Could you check a few things on this model? Use its own coordinates, in mm. A direction names the side the tool comes from. Coordinates: 2 decimals unless noted, no trailing zeros. Loops run counter-clockwise (first coordinate to the right, second up) from the corner with the lowest first, then second, coordinate; pieces in that order, holes last. Notation, with made-up numbers: (-33.75, 82.25) - (12.25, 82.25) arc R22 cw to (12.25, 121.25) - close; hole circle Ø9 at (28.5, 24). An arc over 180 degrees is marked (long way). Use CSV: the item, a comma, the result in double quotes.
from build123d import *

# Parameters (mm, degrees)
CYLINDER001_R           = 0.55
CYLINDER001_DEPTH       = 3.5
CYLINDER_R              = 1.1
CYLINDER_DEPTH          = 3.5
CUBE003_W               = 4
CUBE003_H               = 6
CUBE003_DEPTH           = 9
CUBE003_PLACEMENT_ANGLE = 15
CUBE002_W               = 4
CUBE002_H               = 6
CUBE002_DEPTH           = 8
CUBE002_PLACEMENT_ANGLE = 15
CUBE001_W               = 1.27
CUBE001_H               = 3
CUBE001_DEPTH           = 4
CUBE_W                  = 2.54
CUBE_H                  = 6.2
CUBE_DEPTH              = 8.2


with BuildPart() as cylinder001:
    # cylinder001 → cylinder001 (new body)
    with BuildSketch(Plane(origin=(1.27, 3.1, -3.5), x_dir=(1, 0, 0), z_dir=(0, 0, 1))):
        Circle(CYLINDER001_R)
    extrude(amount=CYLINDER001_DEPTH)


with BuildPart() as cylinder:
    # cylinder → cylinder (new body)
    with BuildSketch(Plane(origin=(1.27, 3.1, 5), x_dir=(1, 0, 0), z_dir=(0, 0, 1))):
        Circle(CYLINDER_R)
    extrude(amount=CYLINDER_DEPTH)


with BuildPart() as cube003:
    # cube003 → cube003 (new body)
    with BuildSketch(Plane.XY):
        with Locations((2, 3)):
            Rectangle(CUBE003_W, CUBE003_H)
    extrude(amount=CUBE003_DEPTH)


with BuildPart() as cube003_1:
    # cube003 placement: moved
    add(cube003.part.moved(Location((-1, -7.244444, 1.941143))).rotate(Axis((-1, -7.244444, 1.941143), (-1, 0, 0)), CUBE003_PLACEMENT_ANGLE))


with BuildPart() as cube002:
    # cube002 → cube002 (new body)
    with BuildSketch(Plane.XY):
        with Locations((2, 3)):
            Rectangle(CUBE002_W, CUBE002_H)
    extrude(amount=CUBE002_DEPTH)


with BuildPart() as cube002_1:
    # cube002 placement: moved
    add(cube002.part.moved(Location((-1, 6.761481, 1.811733))).rotate(Axis((-1, 6.761481, 1.811733), (1, 0, 0)), CUBE002_PLACEMENT_ANGLE))


with BuildPart() as cube001:
    # cube001 → cube001 (new body)
    with BuildSketch(Plane(origin=(0.635, -1, 1), x_dir=(1, 0, 0), z_dir=(0, 0, 1))):
        with Locations((0.635, 1.5)):
            Rectangle(CUBE001_W, CUBE001_H)
    extrude(amount=CUBE001_DEPTH)


with BuildPart() as group:
    # cube → cube (new body)
    with BuildSketch(Plane.XY):
        with Locations((1.27, 3.1)):
            Rectangle(CUBE_W, CUBE_H)
    extrude(amount=CUBE_DEPTH)

    # difference: cut cube001
    add(cube001.part, mode=Mode.SUBTRACT)

    # difference001: cut cube002
    add(cube002_1.part, mode=Mode.SUBTRACT)

    # difference002: cut cube003
    add(cube003_1.part, mode=Mode.SUBTRACT)

    # difference003: cut cylinder
    add(cylinder.part, mode=Mode.SUBTRACT)

    # Group: union cylinder001
    add(cylinder001.part)


solid = group.part
(1) Suppose I cut it at A-A (y = 1). Write out the boundary of the cut face in (x, z) (3 decimals), plus the area to 3 significant figures.
Computed:
outline,"(0, 0) - (2.54, 0) - (2.54, 8.2) - (0, 8.2) - close; hole (0.635, 1) - (1.905, 1) - (1.905, 5) - (0.635, 5) - close"
area,"15.7 mm²"
(2) Will these pins go through, and if not, where does the flat tip stop? pin 1 (1.5 mm diameter, centred on x = 0.5, y = 1, fed in from -Z); pin 2 (0.7 mm diameter, centred on x = 1, y = 3.5, fed in from +Z).
Computed:
pin 1,"stops at z = 0"
pin 2,"stops at z = 5"
(3) Thinking about a two-plate mould opening in X: for faces 1 (the face through (1.252, 5.633, 6.024)), 2 (the face through (0, 3, 4)), 3 (the face through (1, 1, 1)), which applies, +X half, -X half, draft (parallel to the pull), parting line (faces both ways), or undercut?
Computed:
face 1,"draft"
face 2,"-X half"
face 3,"undercut"
(4) Suppose I cut it at D-D (x = 1.1). Write out the boundary of the cut face in (y, z).
Computed:
outline,"(0, 0) - (2.58, 0) - (2.58, -3.5) - (3.62, -3.5) - (3.62, 0) - (6.2, 0) - (6.2, 3.91) - (5.05, 8.2) - (4.19, 8.2) - (4.19, 5) - (2.01, 5) - (2.01, 8.2) - (0.64, 8.2) - (0, 5.8) - (0, 5) - (2, 5) - (2, 1) - (0, 1) - close"
(5) Suppose I cut it at B-B (y = 3.1). Write out the boundary of the cut face in (x, z), plus the area to 3 significant figures.
Computed:
outline,"(0, 0) - (0.72, 0) - (0.72, -3.5) - (1.82, -3.5) - (1.82, 0) - (2.54, 0) - (2.54, 8.2) - (2.37, 8.2) - (2.37, 5) - (0.17, 5) - (0.17, 8.2) - (0, 8.2) - close"
area,"17.6 mm²"
(6) Which directions (+Z, -Z, +X, -X, +Y, -Y) give clear straight access to the entire face, cutting with the end or side of a thin tool? Please do faces 4 (the face through (1, 6.2, 2)), 5 (the face through (1.57, 3.56, -1.77)), 6 (the face through (1.032, 2.026, 6.578)), 7 (the face through (1, 1, 5)).
Computed:
face 4,"+Z, -Z, +X, -X, +Y"
face 5,"-Z"
face 6,"+Z"
face 7,"-Y"
(7) Suppose I cut it at C-C (z = 3). Write out the boundary of the cut face in (x, y) (3 decimals), plus the area to 3 significant figures.
Computed:
outline,"(0, 0) - (0.635, 0) - (0.635, 2) - (1.905, 2) - (1.905, 0) - (2.54, 0) - (2.54, 6.2) - (0, 6.2) - close"
area,"13.2 mm²"
(8) Please list where these lines run through material, in increasing order: line 1 (Z direction, x = 1.25, y = 1.5); line 2 (X direction, y = 3.1, z = 5.9); line 3 (X direction, y = 0.5, z = 4.5) (3 decimals).
Computed:
line 1,"z = 0 to 1, 5 to 8.2"
line 2,"x = 0 to 0.17, 2.37 to 2.54"
line 3,"x = 0 to 0.635, 1.905 to 2.54"
